Check sheet for the modelled part. Datum: model origin and axes. Units: mm. A direction names the side the tool comes from. Round coordinates to 2 decimals unless told otherwise and drop trailing zeros. Write each loop counter-clockwise with the first axis right and the second up, starting at its lowest first coordinate (ties: lowest second). Pieces come first, ordered by that corner, then holes. Notation, with made-up numbers: M 66.5,59.5 L 100.5,59.5 A23 ccw 100.5,82.5 Z; hole C -11.75,36 d3. An arc over 180 degrees is marked long. One line per item, written item: value.
from build123d import *

# Parameters (mm, degrees)
BOSS_EXTRUDE1_DEPTH     = 1540
CUT_EXTRUDE1_DEPTH      = 47886.152097935
CUT_EXTRUDE1_DEPTH_BACK = 47886.152097935
SKETCH2_R               = 3.500000003
SKETCH2_R_2             = 3.5
SKETCH3_R               = 3.5
CUT_EXTRUDE2_DEPTH      = 47886.152097935
LPATTERN1_COUNT         = 11
LPATTERN1_PITCH         = 149
SKETCH4_R               = 3.500000003
CUT_EXTRUDE3_DEPTH      = 47886.152097935
LPATTERN2_COUNT         = 11
LPATTERN2_PITCH         = 150


with BuildPart() as part:
    # Sketch1 → Boss-Extrude1 (new body)
    with BuildSketch(Plane.XY):
        Polygon((47860.381031815, 20322.146461628), (47838.954087292, 20322.146461628), (47798.381031816, 20333.016781299), (47757.807976339, 20322.146461628), (47733.381031815, 20322.146461628), (47719.858070247, 20318.522994997), (47719.590121055, 20319.522994997), (47733.113082623, 20323.146461628), (47757.676337852, 20323.146461628), (47798.381031816, 20334.052049839), (47839.085725779, 20323.146461628), (47860.381031815, 20323.146461628), align=None)
    extrude(amount=BOSS_EXTRUDE1_DEPTH)

    # Sketch2 → Cut-Extrude1 (cut, two sides: drawn at the far end of the back side and taken through both)
    with BuildSketch(Plane(origin=(0, 20323.146461628, 0), x_dir=(1, 0, 0), z_dir=(0, 1, 0)).offset(-CUT_EXTRUDE1_DEPTH_BACK)):
        with Locations(Location((47798.381031816, -20, 0), (0, 0, 90))):
            Circle(SKETCH2_R)
        with Locations(Location((47798.381031816, -70, 0), (0, 0, 90))):
            Circle(SKETCH2_R)
        with Locations(Location((47798.381031818, -1470, 0), (0, 0, 90.000000047))):
            Circle(SKETCH2_R_2)
        with Locations(Location((47798.381031818, -1520, 0), (0, 0, 90.000000047))):
            Circle(SKETCH2_R_2)
    extrude(amount=CUT_EXTRUDE1_DEPTH + CUT_EXTRUDE1_DEPTH_BACK, mode=Mode.SUBTRACT)

    # Sketch3 → Cut-Extrude2 (cut, symmetric)
    with BuildSketch(Plane(origin=(0, 20323.146461628, 0), x_dir=(1, 0, 0), z_dir=(0, 1, 0))):
        with Locations(Location((47851.381031815, -25, 0), (0, 0, 270))):
            Circle(SKETCH3_R)
    cut_extrude2 = extrude(amount=CUT_EXTRUDE2_DEPTH, both=True, mode=Mode.SUBTRACT)

    # LPattern1: Cut-Extrude2 ×11
    with Locations(*[(0, 0, i * LPATTERN1_PITCH) for i in range(1, LPATTERN1_COUNT)]):
        add(cut_extrude2, mode=Mode.SUBTRACT)

    # Sketch4 → Cut-Extrude3 (cut, symmetric)
    with BuildSketch(Plane(origin=(0, 20323.146461628, 0), x_dir=(1, 0, 0), z_dir=(0, 1, 0))):
        with Locations(Location((47744.381031816, -1520, 0), (0, 0, 90))):
            Circle(SKETCH4_R)
    cut_extrude3 = extrude(amount=CUT_EXTRUDE3_DEPTH, both=True, mode=Mode.SUBTRACT)

    # LPattern2: Cut-Extrude3 ×11
    with Locations(*[(0, 0, -i * LPATTERN2_PITCH) for i in range(1, LPATTERN2_COUNT)]):
        add(cut_extrude3, mode=Mode.SUBTRACT)


solid = part.part
Q1. Sectioned sample at A-A on z = 272.5. Enter the section's corners in (x, y), and give its area (3 significant figures).
Completed:
outline: M 47719.59,20319.52 L 47719.86,20318.52 L 47733.38,20322.15 L 47757.81,20322.15 L 47798.38,20333.02 L 47838.95,20322.15 L 47860.38,20322.15 L 47860.38,20323.15 L 47839.09,20323.15 L 47798.38,20334.05 L 47757.68,20323.15 L 47733.11,20323.15 Z
area: 144 mm^2
Q2. Draft check along X on faces 1 (the flat face through (47745, 20323.146, 759)), 2 (the flat face through (47818.952, 20327.506, 759.22)), 3 (the flat face through (47818.448, 20328.676, 759.22)). Enter one of: pulls with the +X half, pulls with the -X half, needs draft (parallel to the pull), parting line crosses it, or undercut.
Completed:
face 1: needs draft
face 2: undercut
face 3: pulls with the +X half
Q3. Depth check by flat-ended pin: P1, Ø7.5, axis at x = 47741.5, z = 938.5, coming from the +Y side; P2, Ø4, axis at x = 47851.38, z = 323, coming from the -Y side; P3, Ø8, axis at x = 47744.38, z = 1370, coming from the -Y side. Enter the tip coordinate at first touch or a pass-through.
Completed:
P1: y = 20323.15
P2: through
P3: y = 20322.15
Q4. Scan lines: line 1 (Y direction, x = 47848.5, z = 442.5); line 2 (Y direction, x = 47732.5, z = 238). Record each from-to range of solid material in increasing order. Write a range as [from, to].
Completed:
line 1: [20322.15, 20323.15]
line 2: [20321.91, 20322.98]
Q5. Access from +Z, -Z, +X, -X, +Y, -Y to the whole of each face (thin tool, end or side, straight path). Record for faces 4 (the flat face through (47746, 20322.146, 759)), 5 (the flat face through (47778.38, 20327.66, 759.22)), 6 (the flat face through (47777.74, 20328.52, 759.22)).
Completed:
face 4: +Z, -Z, +X, -Y
face 5: +Z, -Z, -Y
face 6: +Z, -Z, -X, +Y
Q6. Sectioned sample at B-B on y = 20326.75. Enter the section's corners in (x, z), and give its area (3 significant figures).
Completed:
outline: M 47771.13,0 L 47774.99,0 L 47774.99,1540 L 47771.13,1540 Z; M 47821.77,0 L 47825.64,0 L 47825.64,1540 L 47821.77,1540 Z
area: 11,900 mm^2
